Could you check a few things on this model? Use its own coordinates, in mm. Face numbers are marked on the shaded views. A direction names the side the tool comes from. Give positions to 0.01 mm unless a question says otherwise; leave off trailing zeros. Write each loop counter-clockwise with the first axis right and the second up, starting at its lowest first coordinate (ties: lowest second). Pieces come first, ordered by that corner, then holes. Notation, with made-up numbers: M 15,21.5 L 46,21.5 A34 ccw 46,54.5 Z; hole C 25,6 d11. An arc over 180 degrees is marked long. Write each question's results on one line, items separated by ' | '. Start each with the question number.
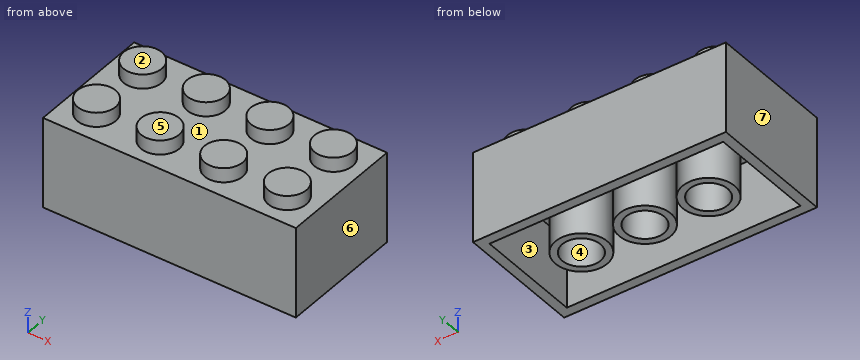
from build123d import *

# Parameters (mm, degrees)
F0_W     = 807.72
F0_H     = 401.32
F1_DEPTH = 289.56
F2_R     = 60.96
F3_DEPTH = 45.72
F4_W     = 746.76
F4_H     = 340.36
F5_DEPTH = 218.44
F6_R     = 82.677
F6_R_2   = 60.96
F7_DEPTH = 218.44


with BuildPart() as f1:
    # F0 (on Top) → F1 (new body)
    with BuildSketch(Plane.XY):
        Rectangle(F0_W, F0_H)
    extrude(amount=F1_DEPTH)

    # F2 (on face) → F3 (join)
    with BuildSketch(Plane.XY.offset(289.56)):
        with Locations((-304.8, -101.6)):
            Circle(F2_R)
        with Locations((-304.8, 101.6)):
            Circle(F2_R)
        with Locations((-101.6, 101.6)):
            Circle(F2_R)
        with Locations((-101.6, -101.6)):
            Circle(F2_R)
        with Locations((101.6, -101.6)):
            Circle(F2_R)
        with Locations((101.6, 101.6)):
            Circle(F2_R)
        with Locations((304.8, 101.6)):
            Circle(F2_R)
        with Locations((304.8, -101.6)):
            Circle(F2_R)
    extrude(amount=F3_DEPTH)

    # F4 (on face) → F5 (cut)
    with BuildSketch(Plane(origin=(0, 0, 0), x_dir=(1, 0, 0), z_dir=(0, 0, -1))):
        Rectangle(F4_W, F4_H)
    extrude(amount=-F5_DEPTH, mode=Mode.SUBTRACT)

    # F6 (on face) → F7 (join)
    with BuildSketch(Plane(origin=(0, 0, 218.44), x_dir=(1, 0, 0), z_dir=(0, 0, -1))):
        with Locations((-203.2, 0)):
            Circle(F6_R)
        with Locations((-203.2, 0)):
            Circle(F6_R_2, mode=Mode.SUBTRACT)
        Circle(F6_R)
        Circle(F6_R_2, mode=Mode.SUBTRACT)
        with Locations((203.2, 0)):
            Circle(F6_R)
        with Locations((203.2, 0)):
            Circle(F6_R_2, mode=Mode.SUBTRACT)
    extrude(amount=F7_DEPTH)


solid = f1.part
Q1. If we section it at B-B (x = 0): Please give me the cut outline in (y, z).
Q2. If we section it at D-D (x = -304.8): Please give me the cut outline in (y, z), plus the area to 3 significant figures.
Q3. Please list where these lines run through material, in increasing order: line 1 (Y direction, x = 0, z = 91); line 2 (X direction, y = 65, z = 94.5); line 3 (Y direction, x = -5, z = 93). Write a range as [from, to].
Q4. For the marked faces 1, 2 and 3, which set-ups out of +Z, -Z, +X, -X, +Y, -Y let a thin tool reach every point of the face, with its end or its side?
Q5. If we section it at A-A (z = 118): Please give me the cut outline in (x, y), plus the area to 3 significant figures.
Q6. I'm going to push a flat-ended pin straight in: P1, Ø4, axis at x = 312.5, y = 154.5, coming from the -Z side. Where does the tip first touch, or does it pass through?
Q7. If we mould it in two halves opening along X, with no side actions, what happens to the marked faces 4, 5, 6 and 7? For each: pulls with the +X half, pulls with the -X half, needs draft (parallel to the pull), parting line crosses it, or undercut.
Q8. If we section it at C-C (y = -101.6): Please give me the cut outline in (x, z).
Determined:
1) outline: M -200.66,0 L -170.18,0 L -170.18,218.44 L -82.68,218.44 L -82.68,0 L -60.96,0 L -60.96,218.44 L 60.96,218.44 L 60.96,0 L 82.68,0 L 82.68,218.44 L 170.18,218.44 L 170.18,0 L 200.66,0 L 200.66,289.56 L -200.66,289.56 Z
2) outline: M -200.66,0 L -170.18,0 L -170.18,218.44 L 170.18,218.44 L 170.18,0 L 200.66,0 L 200.66,289.56 L 162.56,289.56 L 162.56,335.28 L 40.64,335.28 L 40.64,289.56 L -40.64,289.56 L -40.64,335.28 L -162.56,335.28 L -162.56,289.56 L -200.66,289.56 Z | area: 53,000 mm²
3) line 1: y = [-200.66, -170.18], [-82.68, -60.96], [60.96, 82.68], [170.18, 200.66] | line 2: x = [-403.86, -373.38], [-254.29, -152.11], [-51.09, 51.09], [152.11, 254.29], [373.38, 403.86] | line 3: y = [-200.66, -170.18], [-82.53, -60.75], [60.75, 82.53], [170.18, 200.66]
4) face 1: +Z | face 2: +Z, +X, -X, +Y, -Y | face 3: -Z
5) outline: M -403.86,-200.66 L 403.86,-200.66 L 403.86,200.66 L -403.86,200.66 Z; C -203.2,0 d165.35; C 0,0 d165.35; C 203.2,0 d165.35; hole M -373.38,-170.18 L 373.38,-170.18 L 373.38,170.18 L -373.38,170.18 Z; hole C -203.2,0 d121.92; hole C 0,0 d121.92; hole C 203.2,0 d121.92 | area: 99,400 mm²
6) P1: stops at z = 218.44
7) face 4: undercut | face 5: needs draft | face 6: pulls with the +X half | face 7: pulls with the -X half
8) outline: M -403.86,0 L -373.38,0 L -373.38,218.44 L 373.38,218.44 L 373.38,0 L 403.86,0 L 403.86,289.56 L 365.76,289.56 L 365.76,335.28 L 243.84,335.28 L 243.84,289.56 L 162.56,289.56 L 162.56,335.28 L 40.64,335.28 L 40.64,289.56 L -40.64,289.56 L -40.64,335.28 L -162.56,335.28 L -162.56,289.56 L -243.84,289.56 L -243.84,335.28 L -365.76,335.28 L -365.76,289.56 L -403.86,289.56 Z
